CAD build for the part. Positions are in the model's coordinates, mm. A direction names the side the tool comes from. Round coordinates to 2 decimals unless told otherwise and drop trailing zeros. Loops run counter-clockwise (first coordinate to the right, second up) from the corner with the lowest first, then second, coordinate; pieces in that order, holes last. Notation, with made-up numbers: M 63,74 L 92,74 A25 ccw 92,94 Z; hole C 25.25,23 d3. An arc over 180 degrees is marked long. One line per item, written item: value. Start each with the question number.
from build123d import *
from OCP.BRepFilletAPI import BRepFilletAPI_MakeChamfer

# Parameters (mm, degrees)
BOSS_EXTRUDE1_DEPTH = 30
HOLE1_D             = 5.4
HOLE1_DEPTH         = 12.35
HOLE1_CBORE_D       = 6.2
HOLE1_CBORE_DEPTH   = 1
CHAMFER1_SIZE       = 1
CHAMFER1_SIZE_2     = 0.4


with BuildPart() as part:
    # Sketch1 → Boss-Extrude1 (new body)
    with BuildSketch(Plane.XY):
        Polygon((-7.3, 0.3), (-7.3, 7.875735931), (-13.3, 13.875735931), (-13.3, 16.3), (13.3, 16.3), (13.3, 13.875735931), (7.3, 7.875735931), (7.3, 0.3), (23, 0.3), (23, 28.65), (-23, 28.65), (-23, 0.3), align=None)
    extrude(amount=BOSS_EXTRUDE1_DEPTH)

    # Hole1
    with Locations(Plane(origin=(0, 28.65, 0), x_dir=(1, 0, 0), z_dir=(0, 1, 0))):
        with Locations((-7.5, -6.35), (7.5, -6.35), (0, -20)):
            CounterBoreHole(HOLE1_D / 2, HOLE1_CBORE_D / 2, HOLE1_CBORE_DEPTH, depth=HOLE1_DEPTH)

    # Chamfer1
    chamfer1_edges_1 = [part.edges().sort_by_distance(p)[0] for p in [
        (-3.1, 27.65, 20),
    ]]
    chamfer1_side_1 = [part.faces().sort_by_distance(p)[0] for p in [
        (-3.1, 27.658, 20),
    ]]
    chamfer1_edges_2 = [part.edges().sort_by_distance(p)[0] for p in [
        (4.4, 27.65, 6.35),
    ]]
    chamfer1_side_2 = [part.faces().sort_by_distance(p)[0] for p in [
        (4.4, 27.658, 6.35),
    ]]
    chamfer1_edges_3 = [part.edges().sort_by_distance(p)[0] for p in [
        (-10.6, 27.65, 6.35),
    ]]
    chamfer1_side_3 = [part.faces().sort_by_distance(p)[0] for p in [
        (-10.6, 27.658, 6.35),
    ]]
    chamfer1 = BRepFilletAPI_MakeChamfer(part.part.solid().wrapped)
    for e in chamfer1_edges_1:
        chamfer1.Add(CHAMFER1_SIZE - 0.0001, CHAMFER1_SIZE_2 - 0.0001, e.wrapped, chamfer1_side_1[0].wrapped)
    for e in chamfer1_edges_2:
        chamfer1.Add(CHAMFER1_SIZE - 0.0001, CHAMFER1_SIZE_2 - 0.0001, e.wrapped, chamfer1_side_2[0].wrapped)
    for e in chamfer1_edges_3:
        chamfer1.Add(CHAMFER1_SIZE - 0.0001, CHAMFER1_SIZE_2 - 0.0001, e.wrapped, chamfer1_side_3[0].wrapped)
    add(Compound.cast(chamfer1.Shape()), mode=Mode.REPLACE)  # a hair under: the kernel refuses the full size


solid = part.part
(1) Which spindle directions (+Z, -Z, +X, -X, +Y, -Y) get a long thin tool onto all of the face, cutting with end or side? Do faces 5 (the flat face through (-13.3, 15, 15)), 6 (the flat face through (7.3, 4, 15)), 7 (the cylindrical face through (0.351, 21.896, 17.323)). Say none if no direction does.
(2) Slice it at C-C, the plane y = 11. List the corners of the cut face in (x, z), and give its area (3 significant figures).
(3) Probe L1, parallel to X at y = 23, z = 6.35; L2, parallel to X at y = 15.75, z = 1.5; L3, parallel to X at y = 2, z = 17.75. List the from-to ranges inside material, lowest first.
(4) Flat gauge pins, fed straight in: P1, Ø5, axis at x = 0, z = 20, coming from the -Y side; P2, Ø3, axis at x = 7.5, z = 6.35, coming from the +Y side; P3, Ø8, axis at x = 1.5, z = 26, coming from the -Y side; P4, Ø3.5, axis at x = 7.5, z = 6.35, coming from the +Y side. Where does each tip first touch, or does it go through?
(5) Slice it at A-A, the plane z = 6.35. Count the separate pieces of the cut face and the enclosed holes in it, and give its area (3 significant figures).
(6) Slice it at D-D, the plane y = 18.5. List the corners of the cut face in (x, z), and give its area (3 significant figures).
(7) Mould opens along X. For faces 1 (the flat face through (-23, 15, 15)), 2 (the flat face through (15, 0.3, 15)), 3 (the cylindrical face through (-10.075, 21.896, 5.539)), 4 (the flat face through (23, 14, 15)) say: pulls with the +X half, pulls with the -X half, needs draft (parallel to the pull), parting line crosses it, or undercut.
Check result:
1. face 5: +Z, -Z
1. face 6: +Z, -Z, -Y
1. face 7: +Y, -Y
2. outline: M -23,0 L -10.42,0 L -10.42,30 L -23,30 Z; M 10.42,0 L 23,0 L 23,30 L 10.42,30 Z
2. area: 755 mm^2
3. L1: x = -23 to -10.2, -4.8 to 4.8, 10.2 to 23
3. L2: x = -23 to -13.3, 13.3 to 23
3. L3: x = -23 to -7.3, 7.3 to 23
4. P1: passes through
4. P2: stops at y = 9.58
4. P3: stops at y = 16.3
4. P4: stops at y = 9.83
5. separate pieces: 3
5. enclosed holes: 0
5. area: 871 mm^2
6. outline: M -23,0 L 23,0 L 23,30 L -23,30 Z; hole C -7.5,6.35 d5.4; hole C 0,20 d5.4; hole C 7.5,6.35 d5.4
6. area: 1,310 mm^2
7. face 1: pulls with the -X half
7. face 2: needs draft
7. face 3: undercut
7. face 4: pulls with the +X half
